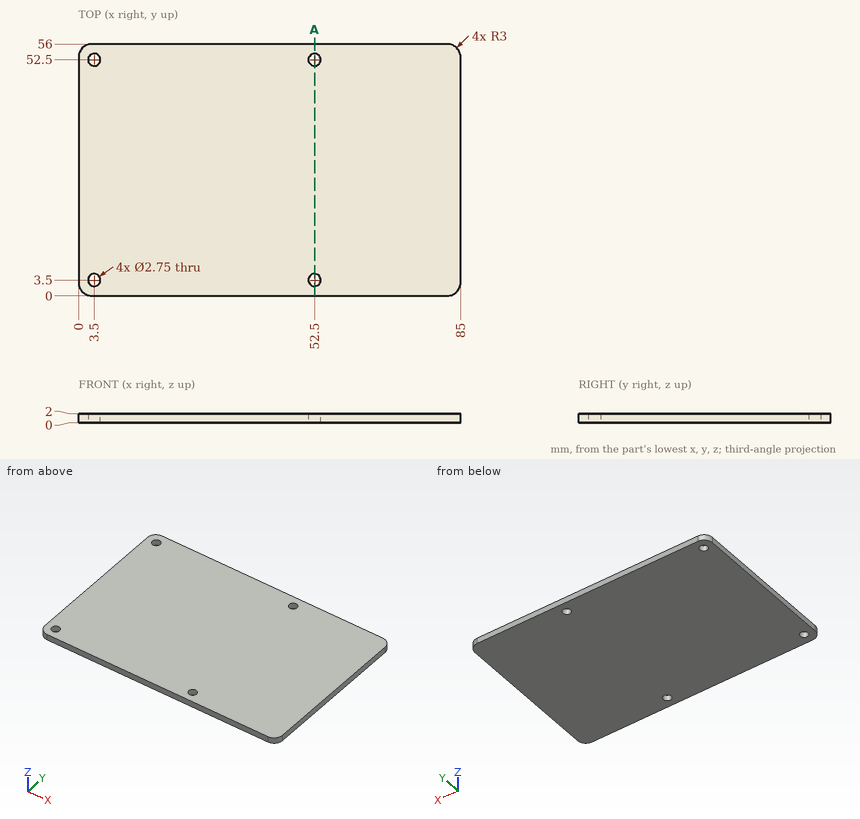
For this review, use the dimensioned drawing (mm, ordinates from the lowest corner) and the shaded views. Give positions to 0.01 mm unless a question says otherwise; leave off trailing zeros. Order: outer loops, then holes, each group sorted by start corner. A loop starts at its lowest first (then second) coordinate and runs counter-clockwise, first axis right, second up. Notation, with made-up numbers: M 63.5,59.25 L 77.5,59.25 A29 cw 77.5,83.25 Z; hole C 74,-37 d11. An arc over 180 degrees is marked long. Use one line per item in the form item = value. Start each with the question number.
Item 1: Insertion check: pin 1 Ø12 at (x, y) = (62.5, 16.5) entering from -Z. The pin has a flat end and moves straight along its axis. Give the tip position at first contact, or say it passes through.
Item 2: To check wall thickness, follow line 1 along Y through (x, z) = (52.5, 0.6) (3 decimals); line 2 along X through (y, z) = (52.5, 1.35) (3 decimals); line 3 along X through (y, z) = (53.5, 1.75). State the ranges of each line that lie inside material, in increasing order. Write a range as from..to.
Item 3: We need section A-A on x = 52.5. Give the boundary of the cut face in (y, z) (3 decimals).
Completed:
q1.pin_1 = 0
q2.line_1 = 0..2.125, 4.875..51.125, 53.875..56
q2.line_2 = 0..2.125, 4.875..51.125, 53.875..85
q2.line_3 = 0.04..2.56, 4.44..51.56, 53.44..84.96
q3.outline = M 0,0 L 2.125,0 L 2.125,2 L 0,2 Z; M 4.875,0 L 51.125,0 L 51.125,2 L 4.875,2 Z; M 53.875,0 L 56,0 L 56,2 L 53.875,2 Z
